```python
from build123d import *

# Parameters (mm, degrees)
F0_R     = 304.8
F1_DEPTH = 304.8
F2_R     = 190.498437
F3_DEPTH = 645.16
F4_R     = 50.8
F6_DEPTH = 66.04


with BuildPart() as f1:
    # F0 (on Front) → F1 (new body)
    with BuildSketch(Plane.XZ):
        Circle(F0_R)
    extrude(amount=F1_DEPTH)

    # F2 (on face) → F3 (cut)
    with BuildSketch(Plane(origin=(0, 0, 0), x_dir=(-1, 0, 0), z_dir=(0, 1, 0))):
        Circle(F2_R)
    extrude(amount=-F3_DEPTH, mode=Mode.SUBTRACT)

    # F4
    f4_edges = [f1.edges().sort_by_distance(p)[0] for p in [
        (-304.8, -304.8, 0),
        (-304.8, 0, 0),
    ]]
    fillet(f4_edges, radius=F4_R)

    # F5 (on face) → F6 (join)
    with BuildSketch(Plane(origin=(0, 0, 0), x_dir=(-1, 0, 0), z_dir=(0, 1, 0))):
        Polygon((151.48038, -156.267236), (151.48038, -168.967236), (163.558798, -172.891752), (171.023671, -162.617236), (163.558798, -152.342721), align=None)
    extrude(amount=F6_DEPTH)


solid = f1.part
```
Read the model definition and answer for the solid it produces. Units are mm, in the model's axes. Give positions to 0.01 mm unless a question says otherwise; leave off trailing zeros. Order: outer loops, then holes, each group sorted by start corner. A loop starts at its lowest first (then second) coordinate and runs counter-clockwise, first axis right, second up. Notation, with made-up numbers: (-11.5, 38.25) -> (46.5, 38.25) arc R21 ccw to (46.5, 75.25) -> close; hole circle Ø11 at (61.25, 45.25). An arc over 180 degrees is marked (long way). Write item = value, one per line.
1. A cutting plane is placed at B-B, the plane x = 0. Write down the section's boundary in (y, z), and give its area (3 significant figures).
Numbers:
outline = (-304.8, -254) arc R50.8 ccw to (-254, -304.8) -> (-50.8, -304.8) arc R50.8 ccw to (0, -254) -> (0, -190.5) -> (-304.8, -190.5) -> close; (-304.8, 190.5) -> (0, 190.5) -> (0, 254) arc R50.8 ccw to (-50.8, 304.8) -> (-254, 304.8) arc R50.8 ccw to (-304.8, 254) -> close
area = 67,500 mm²
2. The mould has two halves that part along Z. Classify faces 1 (the face through (36, -304.8, 189)), 2 (the face through (-241.879, -150.978, -185.466)), 3 (the face through (151.17, -150.27, -115.92)): +Z half, -Z half, draft (parallel to the pull), parting line (faces both ways), or undercut.
Numbers:
face_1 = draft
face_2 = parting line
face_3 = undercut
3. Given pin 1 (5 mm diameter, centred on y = -127.5, z = -23, fed in from +X); pin 2 (10 mm diameter, centred on y = 18, z = -163, fed in from +X); pin 3 (1 mm diameter, centred on x = 108.5, y = -258, fed in from +Z), each flat-ended and moving along its own axis, determine where each tip first touches the part or whether it passes through.
Numbers:
pin_1 = 304.11
pin_2 = -151.48
pin_3 = 284.86
4. A cutting plane is placed at C-C, the plane y = -201. Write down the section's boundary in (x, z), and give its area (3 significant figures).
Numbers:
outline = circle Ø609.6 at (0, 0); hole circle Ø381 at (0, 0)
area = 178,000 mm²
5. A cutting plane is placed at A-A, the plane z = 0. Write down the section's boundary in (x, y), and give its area (3 significant figures).
Numbers:
outline = (-304.8, -254) arc R50.8 ccw to (-254, -304.8) -> (-190.5, -304.8) -> (-190.5, 0) -> (-254, 0) arc R50.8 ccw to (-304.8, -50.8) -> close; (190.5, -304.8) -> (254, -304.8) arc R50.8 ccw to (304.8, -254) -> (304.8, -50.8) arc R50.8 ccw to (254, 0) -> (190.5, 0) -> close
area = 67,500 mm²
6. A cutting plane is placed at D-D, the plane y = -14.5. Write down the section's boundary in (x, z), and give its area (3 significant figures).
Numbers:
outline = circle Ø579.08 at (0, 0); hole circle Ø381 at (0, 0)
area = 149,000 mm²
7. Straight lines are drawn through the part: line 1 along Z through (x, y) = (0, -69); line 2 along Y through (x, z) = (-123, -216.5); line 3 along X through (y, z) = (-253.5, 148). For each, find the intervals that lie inside material, in ascending order.
Numbers:
line_1 = -304.8 to -190.5, 190.5 to 304.8
line_2 = -304.8 to 0
line_3 = -266.46 to -119.94, 119.94 to 266.46
